from build123d import *

# Parameters (mm, degrees)
SKETCH_1_R          = 3
EXTRUDE_1_DEPTH     = 17.5
SKETCH_2_R          = 4
EXTRUDE_2_DEPTH     = 2
EXTRUDE_START       = 2
SKETCH_3_R          = 4
EXTRUDE_3_DEPTH     = 2
SKETCH_4_R          = 3
EXTRUDE_4_DEPTH     = 20
SKETCH_5_R          = 4
EXTRUDE_5_DEPTH     = 2
SKETCH_7_R          = 4
CUT_EXTRUDE_1_DEPTH = 16
SKETCH_8_R          = 4
EXTRUDE_6_DEPTH     = 2


with BuildPart() as part:
    # 草图1 → 凸台-拉伸1 (new body)
    with BuildSketch(Plane.XY):
        Circle(SKETCH_1_R)
    extrude(amount=EXTRUDE_1_DEPTH)

    # 草图2 → 凸台-拉伸2 (add)
    with BuildSketch(Plane(origin=(0, 0, 0), x_dir=(-1, 0, 0), z_dir=(0, 0, -1))):
        Circle(SKETCH_2_R)
    extrude(amount=EXTRUDE_2_DEPTH)

    # 草图3 → 凸台-拉伸3 (add)
    with BuildSketch(Plane.XY.offset(17.5).offset(EXTRUDE_START)):
        with Locations(Location((0, 0, 0), (0, 0, 180))):
            Circle(SKETCH_3_R)
    extrude(amount=-EXTRUDE_3_DEPTH)

    # 草图4 → 凸台-拉伸4 (add)
    with BuildSketch(Plane.XY.offset(19.5)):
        Circle(SKETCH_4_R)
    extrude(amount=EXTRUDE_4_DEPTH)

    # 草图5 → 凸台-拉伸5 (add)
    with BuildSketch(Plane.XY.offset(39.5).offset(EXTRUDE_START)):
        with Locations(Location((0, 0, 0), (0, 0, 180))):
            Circle(SKETCH_5_R)
    extrude(amount=-EXTRUDE_5_DEPTH)

    # 草图7 → 切除-拉伸1 (cut)
    with BuildSketch(Plane.XY.offset(41.5)):
        with Locations(Location((0, 0, 0), (0, 0, 180))):
            Circle(SKETCH_7_R)
    extrude(amount=-CUT_EXTRUDE_1_DEPTH, mode=Mode.SUBTRACT)

    # 草图8 → 凸台-拉伸6 (add)
    with BuildSketch(Plane.XY.offset(25.5).offset(EXTRUDE_START)):
        with Locations(Location((0, 0, 0), (0, 0, 180))):
            Circle(SKETCH_8_R)
    extrude(amount=-EXTRUDE_6_DEPTH)


solid = part.part
Source: CAD feature listing. Evaluate the final solid. Frame: model axes, mm. A direction names the side the tool comes from. Give positions to 0.01 mm unless a question says otherwise; leave off trailing zeros. Order: outer loops, then holes, each group sorted by start corner. A loop starts at its lowest first (then second) coordinate and runs counter-clockwise, first axis right, second up. Notation, with made-up numbers: (-27.5, 40) -> (-14.5, 40) arc R21 cw to (-14.5, 75) -> close; hole circle Ø8 at (63, 61.25). An arc over 180 degrees is marked (long way). Use a Markdown table: item, result.
1) Reachability of faces 5 (the flat face through (0, 0, -2)), 6 (the flat face through (-1, 3, 0)) from +Z, -Z, +X, -X, +Y, -Y: full face, straight path, thin tool, end or side. Return the list, or none.
Answer list:
| item | result |
|---|---|
| face 5 | -Z, +X, -X, +Y, -Y |
| face 6 | none |
2) Mould query, pull axis Z, two halves, no side actions, for faces 1 (the flat face through (-1, -3, 25.5)), 2 (the flat face through (0, 0, 27.5)), 3 (the cylindrical face through (-3, 0, 22)), 4 (the cylindrical face through (0.867, -3.905, -0.986)). Classes: +Z half, -Z half, draft (parallel to the pull), parting line (faces both ways), or undercut.
Answer list:
| item | result |
|---|---|
| face 1 | undercut |
| face 2 | +Z half |
| face 3 | undercut |
| face 4 | draft |
3) Ray query, line 1 along Z through (x, y) = (3.25, -1.5); line 2 along X through (y, z) = (1.5, 26.25); line 3 along X through (y, z) = (2.25, -0.25). Return the intervals inside material, ascending. Write a range as [from, to].
Answer list:
| item | result |
|---|---|
| line 1 | [-2, 0], [17.5, 19.5], [25.5, 27.5] |
| line 2 | [-3.71, 3.71] |
| line 3 | [-3.31, 3.31] |
4) Contact query for flat-ended pins moving along their axis: P1, Ø2, axis at x = -3, z = 3, coming from the -Y side; P2, Ø4, axis at y = 2, z = 16, coming from the +X side; P3, Ø3, axis at x = 0, z = 14.5, coming from the +Y side. Output: stop coordinate, or through.
Answer list:
| item | result |
|---|---|
| P1 | y = -2.24 |
| P2 | x = 3.94 |
| P3 | y = 3 |
5) Section query A-A, the plane y = 3.5. Return the cut outline in (x, z), then the cut area to 3 significant figures.
Answer list:
| item | result |
|---|---|
| outline | (-1.94, -2) -> (1.94, -2) -> (1.94, 0) -> (-1.94, 0) -> close; (-1.94, 17.5) -> (1.94, 17.5) -> (1.94, 19.5) -> (-1.94, 19.5) -> close; (-1.94, 25.5) -> (1.94, 25.5) -> (1.94, 27.5) -> (-1.94, 27.5) -> close |
| area | 23.2 mm² |
6) Section query B-B, the plane x = 0. Return the cut outline in (y, z), then the cut area to 3 significant figures.
Answer list:
| item | result |
|---|---|
| outline | (-4, -2) -> (4, -2) -> (4, 0) -> (3, 0) -> (3, 17.5) -> (4, 17.5) -> (4, 19.5) -> (3, 19.5) -> (3, 25.5) -> (4, 25.5) -> (4, 27.5) -> (-4, 27.5) -> (-4, 25.5) -> (-3, 25.5) -> (-3, 19.5) -> (-4, 19.5) -> (-4, 17.5) -> (-3, 17.5) -> (-3, 0) -> (-4, 0) -> close |
| area | 189 mm² |
7) Section query D-D, the plane z = 1. Return the cut outline in (x, y).
Answer list:
| item | result |
|---|---|
| outline | circle Ø6 at (0, 0) |
